Work out the finished part from the listing and answer in its coordinate system (mm). A direction names the side the tool comes from. Round coordinates to 2 decimals unless told otherwise and drop trailing zeros. Write each loop counter-clockwise with the first axis right and the second up, starting at its lowest first coordinate (ties: lowest second). Pieces come first, ordered by that corner, then holes. Notation, with made-up numbers: (60.25, 1.5) - (96.25, 1.5) arc R32 ccw to (96.25, 28.5) - close; hole circle Ø11 at (2.5, -9). An arc over 180 degrees is marked (long way). Answer as a JSON object with one key per item and string values.
```python
from build123d import *

# Parameters (mm, degrees)
SKETCH3_R            = 6.985
BASE_EXTRUDE_DEPTH   = 0.762
SKETCH4_R            = 8.5852
BOSS_EXTRUDE2_DEPTH  = 3.175
FILLET1_R            = 3.175
FILLET1_OF_MIRROR1_R = 3.175
SKETCH5_R            = 2.3749
CUT_EXTRUDE1_DEPTH   = 15.47104687


with BuildPart() as part:
    # Sketch3 → Base-Extrude (new, symmetric)
    with BuildSketch(Plane.XY):
        with Locations(Location((0, 0, 0), (0, 0, 180))):
            Circle(SKETCH3_R)
    extrude(amount=BASE_EXTRUDE_DEPTH, both=True)

    # Sketch4 → Boss-Extrude2 (add)
    with BuildSketch(Plane.XY.offset(0.762)):
        Circle(SKETCH4_R)
    boss_extrude2 = extrude(amount=BOSS_EXTRUDE2_DEPTH)

    # Fillet1
    fillet1_edges = [part.edges().sort_by_distance(p)[0] for p in [
        (-8.5852, 0, 3.937),
    ]]
    fillet(fillet1_edges, radius=FILLET1_R - 0.0001)  # a hair under: the kernel refuses the full size

    # Mirror1: Boss-Extrude2 across plane
    add(boss_extrude2.mirror(Plane.XY))

    # Fillet1 of Mirror1
    fillet1_of_mirror1_edges = [part.edges().sort_by_distance(p)[0] for p in [
        (-8.5852, 0, -3.937),
    ]]
    fillet(fillet1_of_mirror1_edges, radius=FILLET1_OF_MIRROR1_R - 0.0001)  # a hair under: the kernel refuses the full size

    # Sketch5 → Cut-Extrude1 (cut, through all)
    with BuildSketch(Plane.XY.offset(3.937)):
        Circle(SKETCH5_R)
    extrude(amount=-CUT_EXTRUDE1_DEPTH, mode=Mode.SUBTRACT)


solid = part.part
```
Item 1: For faces 5 (the flat face through (2.3, -1.1, -3.937)), 6 (the cylindrical face through (0.909, -6.926, 0.011)), determine the directions among +Z, -Z, +X, -X, +Y, -Y from which every point of the face is accessible in a straight line to the end or side of a thin tool.
Results found:
{"face 5": "-Z, +X, -X, +Y, -Y", "face 6": "none"}
Item 2: Determine the mould class of faces 1 (the flat face through (2.3, -1.1, 3.937)), 2 (the flat face through (2, -7, 0.762)), 3 (the flat face through (2, -7, -0.762)), 4 (the cylindrical face through (-1.75, 1.605, 0.055)) for opening direction Z: pulls with the +Z half, pulls with the -Z half, needs draft (parallel to the pull), parting line crosses it, or undercut.
Results found:
{"face 1": "pulls with the +Z half", "face 2": "undercut", "face 3": "undercut", "face 4": "needs draft"}
Item 3: A cutting plane is placed at C-C (z = 0). Write down the section's boundary in (x, y) (3 decimals), and give its area (3 significant figures).
Results found:
{"outline": "circle Ø13.97 at (0, 0); hole circle Ø4.75 at (0, 0)", "area": "136 mm²"}
Item 4: Consider line 1 along Y through (x, z) = (0, 0.5) (3 decimals); line 2 along Z through (x, y) = (-6.25, -4.75); line 3 along Z through (x, y) = (-2.75, 6.5). Determine where each line is inside the solid, lowest interval first.
Results found:
{"line 1": "-6.985 to -2.375, 2.375 to 6.985", "line 2": "-2.79 to -0.76, 0.76 to 2.79", "line 3": "-3.48 to -0.76, 0.76 to 3.48"}
Item 5: Each of these flat-tipped pins is pushed along its axis until it touches: P1, Ø5, axis at x = 6.5, y = 3.5, coming from the +Z side; P2, Ø2, axis at x = 6, y = 6, coming from the +Z side; P3, Ø3, axis at x = -1.5, z = 2.5, coming from the +Y side; P4, Ø3, axis at x = 5, y = 6, coming from the -Z side. Where does it stop, or does it pass through?
Results found:
{"P1": "z = 3.94", "P2": "z = 3.17", "P3": "y = 8.52", "P4": "z = -3.81"}
Item 6: A cutting plane is placed at D-D (z = -3). Write down the section's boundary in (x, y).
Results found:
{"outline": "circle Ø15.32 at (0, 0); hole circle Ø4.75 at (0, 0)"}
